```python
from build123d import *

# Parameters (mm, degrees)
F0_R     = 2.5
F0_R_2   = 25
F1_DEPTH = 1.5


with BuildPart() as f1:
    # F0 (on Front) → F1 (new body)
    with BuildSketch(Plane.XZ):
        with BuildLine():
            ThreePointArc((0, 5), (1.464466, 1.464466), (5, 0))
            Line((5, 0), (175, 0))
            ThreePointArc((175, 0), (178.535534, 1.464466), (180, 5))
            Line((180, 5), (180, 175))
            ThreePointArc((180, 175), (178.535534, 178.535534), (175, 180))
            Line((175, 180), (5, 180))
            ThreePointArc((5, 180), (1.464466, 178.535534), (0, 175))
            Line((0, 175), (0, 5))
        make_face()
        with BuildLine():
            ThreePointArc((25, 75), (28.086583, 79.619398), (33.535534, 78.535534))
            Line((33.535534, 78.535534), (78.535534, 33.535534))
            ThreePointArc((78.535534, 33.535534), (79.619398, 28.086583), (75, 25))
            Line((75, 25), (30, 25))
            ThreePointArc((30, 25), (26.464466, 26.464466), (25, 30))
            Line((25, 30), (25, 75))
        make_face(mode=Mode.SUBTRACT)
        with Locations((65, 65)):
            Circle(F0_R, mode=Mode.SUBTRACT)
        with BuildLine():
            Line((101.464466, 33.535534), (146.464466, 78.535534))
            ThreePointArc((146.464466, 78.535534), (151.913417, 79.619398), (155, 75))
            Line((155, 75), (155, 30))
            ThreePointArc((155, 30), (153.535534, 26.464466), (150, 25))
            Line((150, 25), (105, 25))
            ThreePointArc((105, 25), (100.380602, 28.086583), (101.464466, 33.535534))
        make_face(mode=Mode.SUBTRACT)
        with Locations((115, 65)):
            Circle(F0_R, mode=Mode.SUBTRACT)
        with Locations((65, 115)):
            Circle(F0_R, mode=Mode.SUBTRACT)
        with BuildLine():
            ThreePointArc((25, 150), (26.464466, 153.535534), (30, 155))
            Line((30, 155), (75, 155))
            ThreePointArc((75, 155), (79.619398, 151.913417), (78.535534, 146.464466))
            Line((78.535534, 146.464466), (33.535534, 101.464466))
            ThreePointArc((33.535534, 101.464466), (28.086583, 100.380602), (25, 105))
            Line((25, 105), (25, 150))
        make_face(mode=Mode.SUBTRACT)
        with Locations((90, 90)):
            Circle(F0_R_2, mode=Mode.SUBTRACT)
        with Locations((115, 115)):
            Circle(F0_R, mode=Mode.SUBTRACT)
        with BuildLine():
            ThreePointArc((155, 105), (151.913417, 100.380602), (146.464466, 101.464466))
            Line((146.464466, 101.464466), (101.464466, 146.464466))
            ThreePointArc((101.464466, 146.464466), (100.380602, 151.913417), (105, 155))
            Line((105, 155), (150, 155))
            ThreePointArc((150, 155), (153.535534, 153.535534), (155, 150))
            Line((155, 150), (155, 105))
        make_face(mode=Mode.SUBTRACT)
    extrude(amount=F1_DEPTH)


solid = f1.part
```
Build history of the part. All positions in model axes, mm. A direction names the side the tool comes from. Round coordinates to 2 decimals unless told otherwise and drop trailing zeros. Order: outer loops, then holes, each group sorted by start corner. A loop starts at its lowest first (then second) coordinate and runs counter-clockwise, first axis right, second up. Notation, with made-up numbers: (-10.75, 64) - (4.25, 64) arc R13 cw to (4.25, 77) - close; hole circle Ø9 at (-23, 88). An arc over 180 degrees is marked (long way). Use a Markdown table: item, result.
1) Saw through at D-D on y = -0.95. Give the number of separate pieces and of enclosed holes in the cut face, and give its area (3 significant figures).
Recorded:
| item | result |
|---|---|
| separate pieces | 1 |
| enclosed holes | 9 |
| area | 22,900 mm² |
2) Pull direction Z, two halves, no side cores. Call faces 3 (the face through (179, -1, 178)), 4 (the face through (1, -1, 2)), 5 (the face through (26, -1, 153)): pulls with the +Z half, pulls with the -Z half, needs draft (parallel to the pull), parting line crosses it, or undercut.
Recorded:
| item | result |
|---|---|
| face 3 | pulls with the +Z half |
| face 4 | pulls with the -Z half |
| face 5 | undercut |
3) Tool access for faces 1 (the face through (69, -1.5, 111)), 2 (the face through (100.413, -0.74, 28.011)): list every direction of +Z, -Z, +X, -X, +Y, -Y with a clear straight run to the whole face (end or side of a thin tool).
Recorded:
| item | result |
|---|---|
| face 1 | +Z, -Z, +X, -X, -Y |
| face 2 | +Y, -Y |
4) Saw through at B-B on z = 51.5. Write the cut outline in (x, y).
Recorded:
| item | result |
|---|---|
| outline | (0, -1.5) - (25, -1.5) - (25, 0) - (0, 0) - close; (60.57, -1.5) - (119.43, -1.5) - (119.43, 0) - (60.57, 0) - close; (155, -1.5) - (180, -1.5) - (180, 0) - (155, 0) - close |
5) Saw through at C-C on x = 48.5. Write the cut outline in (y, z), and give its area (3 significant figures).
Recorded:
| item | result |
|---|---|
| outline | (-1.5, 0) - (0, 0) - (0, 25) - (-1.5, 25) - close; (-1.5, 63.57) - (0, 63.57) - (0, 116.43) - (-1.5, 116.43) - close; (-1.5, 155) - (0, 155) - (0, 180) - (-1.5, 180) - close |
| area | 154 mm² |
6) Saw through at A-A on x = 90. Write the cut outline in (y, z), and give its area (3 significant figures).
Recorded:
| item | result |
|---|---|
| outline | (-1.5, 0) - (0, 0) - (0, 65) - (-1.5, 65) - close; (-1.5, 115) - (0, 115) - (0, 180) - (-1.5, 180) - close |
| area | 195 mm² |
7) Flat gauge pin, fed straight in: pin 1 Ø4.5 at (x, z) = (65, 115) entering from -Y. Where does the tip first touch, or does it go through?
Recorded:
| item | result |
|---|---|
| pin 1 | passes through |
8) Wall check: L1, parallel to Z at x = 102, y = -0.45; L2, parallel to Z at x = 133, y = -0.9; L3, parallel to X at y = -0.8, z = 59. Give the ranges that are in metal, low to high.
Recorded:
| item | result |
|---|---|
| L1 | z = 0 to 26, 34.07 to 68.07, 111.93 to 145.93, 154 to 180 |
| L2 | z = 0 to 25, 65.07 to 114.93, 155 to 180 |
| L3 | x = 0 to 25, 53.07 to 126.93, 155 to 180 |
